The listing builds one solid part. Answer for the finished solid, in the listing's coordinates (mm). A direction names the side the tool comes from. Round coordinates to 2 decimals unless told otherwise and drop trailing zeros. Write each loop counter-clockwise with the first axis right and the second up, starting at its lowest first coordinate (ties: lowest second). Pieces come first, ordered by that corner, then holes.
(1) Find the intervals of material crossed by probe 1 along Z at (x, y) = (32, 20.5); probe 2 along X at (y, z) = (42, 33.5); probe 3 along Y at (x, z) = (114, -35), in increasing order.
(2) Each of these flat-tipped pins is pushed along its axis until it touches: pin 1 Ø6 at (y, z) = (30, 81.5) entering from -X; pin 2 Ø2 at (x, z) = (30.5, -34) entering from -Y; pin 3 Ø12 at (x, z) = (14, 46.5) entering from +Y. Where does it stop, or does it pass through?
(3) The mould has two halves that part along Z. Classify faces 4 (the face through (-2, 32, 131.25)), 5 (the face through (-115, 64.5, 2)), 6 (the face through (1, 52, 100.85)): +Z half, -Z half, draft (parallel to the pull), parting line (faces both ways), or undercut.
(4) For faces 1 (the face through (1, 52, -100.85)), 2 (the face through (2, 15, -100.85)), 3 (the face through (2, 0, 116)), determine the directions among +Z, -Z, +X, -X, +Y, -Y from which every point of the face is accessible in a straight line to the end or side of a thin tool.
(5) A cutting plane is placed at C-C, the plane x = 19. Give the vertices of the cut face in (y, z), and give its area (3 significant figures).
(6) A cutting plane is placed at B-B, the plane z = -14. Give the vertices of the cut face in (x, y), and give its area (3 significant figures).
(7) A cutting plane is placed at A-A, the plane y = 5. Give the vertices of the cut face in (x, z).
Autodesk Inventor part; units mm, degrees
ref_plane "YZ Plane" through (0, 0, 0) normal (1, 0, 0) x (0, 1, 0)
ref_plane "XZ Plane" through (0, 0, 0) normal (0, 1, 0) x (-1, 0, 0)
ref_plane "XY Plane" through (0, 0, 0) normal (0, 0, 1) x (1, 0, 0)
sketch "Esboço1" plane through (0, 0, 0) normal (0, 1, 0) x (-1, 0, 0)
  line L0 (130.95, 131.25) -> (-130.95, 131.25)
  line L1 (-130.95, 131.25) -> (-130.95, -131.25)
  line L2 (-130.95, -131.25) -> (130.95, -131.25)
  line L3 (130.95, -131.25) -> (130.95, 131.25)
  line L4 (130.95, 131.25) -> (-130.95, -131.25) construction
  line L5 (-130.95, 131.25) -> (130.95, -131.25) construction
  line L6 (-100.55, 100.85) -> (100.55, 100.85)
  line L7 (100.55, 100.85) -> (100.55, -100.85)
  line L8 (100.55, -100.85) -> (-100.55, -100.85)
  line L9 (-100.55, -100.85) -> (-100.55, 100.85)
  line L10 (100.55, 100.85) -> (130.95, 100.85)
  line L11 (-100.55, 100.85) -> (-130.95, 100.85)
  line L12 (100.55, -100.85) -> (130.95, -100.85)
  line L13 (-100.55, -100.85) -> (-130.95, -100.85)
  point P0 (0, 0)
  dimension "d0" = 261.9
  dimension "d1" = 262.5
  dimension "d2" = 30.4
extrude "Extrusão1" add sketch "Esboço1" along normal blind 64.5
extrude "Extrusão2" cut sketch "Esboço1" along normal blind 30.4 contours L3 L12 L7 L10 | L11 L9 L13 L1 | L7 L8 L9 L6
sketch "Esboço2" plane through (0, 64.5, 0) normal (0, 1, 0) x (1, 0, 0)
  line L0 (130.95, 131.25) -> (-130.95, 131.25)
  line L1 (-130.95, 131.25) -> (-130.95, -131.25)
  line L2 (-130.95, -131.25) -> (130.95, -131.25)
  line L3 (130.95, -131.25) -> (130.95, 131.25)
  line L4 (130.95, -131.25) -> (130.95, 131.25)
  line L5 (100.55, 100.85) -> (100.55, -100.85)
  line L6 (100.55, -100.85) -> (-100.55, -100.85)
  line L7 (-100.55, -100.85) -> (-100.55, 100.85)
  line L8 (130.95, 100.85) -> (-130.95, 100.85)
  point P0 (0, 0)
extrude "Extrusão3" cut sketch "Esboço2" against normal blind 25.3 contours L5 L6 L7 L8
sketch "Esboço3" plane through (130.95, 0, -131.25) normal (1, 0, 0) x (0, 0, -1)
  line L0 (-232.1, 30.4) -> (-30.4, 30.4)
  line L1 (-131.25, 30.4) -> (-131.25, 64.5) construction
  line L2 (-262.5, 64.5) -> (0, 64.5)
  line L3 (-232.1, 0) -> (-232.1, 30.4)
  line L4 (-232.1, 30.4) -> (-30.4, 30.4)
  line L5 (-30.4, 30.4) -> (-30.4, 0)
  line L6 (-30.4, 0) -> (0, 0)
  line L7 (0, 0) -> (0, 64.5)
  line L8 (-262.5, 64.5) -> (0, 64.5)
  line L9 (-262.5, 0) -> (-262.5, 64.5)
  line L10 (-262.5, 0) -> (-232.1, 0)
  line L11 (-232.1, 39.2) -> (-30.4, 39.2)
  circle A0 centre (-131.25, 42.7) radius 3.5
  point P0 (-131.25, 0)
  dimension "d9" = 7
sketch "Esboço4" plane through (100.55, 64.5, -100.85) normal (-1, 0, 0) x (0, 0, 1)
  circle A0 centre (100.85, -21.8) radius 3.5
  circle A1 centre (100.85, -10) radius 3.5
  line L0 (232.1, 0) -> (-30.4, 0)
  line L1 (100.85, 0) -> (100.85, -10) construction
  point P0 (100.85, -64.5)
  dimension "d10" = 7
  dimension "d11" = 10
sketch3d "Esboço 3D1"
  line L0 (130.95, 42.7, 0) -> (100.55, 54.5, 0)
sweep "Varredura1" cut profiles "Esboço3" path "Esboço 3D1" contours A0
properties part number "FundoColmeia"
Solutions:
1. probe 1: z = -131.25 to -100.85, 100.85 to 131.25
1. probe 2: x = -130.95 to -100.55, 100.55 to 130.95
1. probe 3: y = 30.4 to 64.5
2. pin 1: stops at x = -130.95
2. pin 2: stops at y = 30.4
2. pin 3: stops at y = 39.2
3. face 4: +Z half
3. face 5: draft
3. face 6: undercut
4. face 1: +Y
4. face 2: +X, -X, -Y
4. face 3: +Z, -Z, +X, -X, -Y
5. outline: (0, -131.25) - (64.5, -131.25) - (64.5, -100.85) - (39.2, -100.85) - (39.2, 100.85) - (64.5, 100.85) - (64.5, 131.25) - (0, 131.25) - (0, 100.85) - (30.4, 100.85) - (30.4, -100.85) - (0, -100.85) - close
5. area: 5,700 mm2
6. outline: (-130.95, 30.4) - (130.95, 30.4) - (130.95, 64.5) - (100.55, 64.5) - (100.55, 39.2) - (-100.55, 39.2) - (-100.55, 64.5) - (-130.95, 64.5) - close
6. area: 3,840 mm2
7. outline: (-130.95, -131.25) - (130.95, -131.25) - (130.95, -100.85) - (-130.95, -100.85) - close; (-130.95, 100.85) - (130.95, 100.85) - (130.95, 131.25) - (-130.95, 131.25) - close
